from build123d import *

# Parameters (mm, degrees)
F0_W     = 50.8
F0_H     = 400.05
F0_W_2   = 23.167712307
F0_H_2   = 133.35
F0_H_3   = 88.3720067978
F0_H_4   = 368.3754058838
F0_H_5   = 197.3025873184
F0_H_6   = 25.4
F0_H_7   = 431.8
F1_DEPTH = 25.4


with BuildPart() as f1:
    # F0 (on Top) → F1 (new body)
    with BuildSketch(Plane.XY):
        with Locations((0, 200.025)):
            Rectangle(F0_W, F0_H)
        with Locations((-36.9838561535, 466.725)):
            Rectangle(F0_W_2, F0_H_2)
        with Locations((0, 466.725)):
            Rectangle(F0_W, F0_H_2)
        with Locations((36.9838561535, 466.725)):
            Rectangle(F0_W_2, F0_H_2)
        with Locations((-36.9838561535, 577.5860033989)):
            Rectangle(F0_W_2, F0_H_3)
        with Locations((36.9838561535, 577.5860033989)):
            Rectangle(F0_W_2, F0_H_3)
        Polygon((-48.567712307, 621.7720067978), (-25.4, 621.7720067978), (-25.4, 990.1474126816), (-152.4, 990.1474126816), (-152.4, 533.4), (-48.567712307, 533.4), align=None)
        with Locations((0, 805.9597097397)):
            Rectangle(F0_W, F0_H_4)
        Polygon((25.4, 990.1474126816), (25.4, 621.7720067978), (48.567712307, 621.7720067978), (48.567712307, 533.4), (152.4, 533.4), (152.4, 990.1474126816), align=None)
        with Locations((0, 1088.7987063408)):
            Rectangle(F0_W, F0_H_5)
        Polygon((-196.85, 1187.45), (-25.4, 1187.45), (-25.4, 1212.85), (-196.85, 1212.85), (-196.85, 1384.3), (-222.25, 1384.3), (-222.25, 1149.35), (-196.85, 1149.35), align=None)
        with Locations((0, 1200.15)):
            Rectangle(F0_W, F0_H_6)
        Polygon((25.4, 1212.85), (25.4, 1187.45), (196.85, 1187.45), (196.85, 1149.35), (222.25, 1149.35), (222.25, 1384.3), (196.85, 1384.3), (196.85, 1212.85), align=None)
        with Locations((0, 1428.75)):
            Rectangle(F0_W, F0_H_7)
        with Locations((0, 577.5860033989)):
            Rectangle(F0_W, F0_H_3)
    extrude(amount=F1_DEPTH)


solid = f1.part
Read the model definition and answer for the solid it produces. Units are mm, in the model's axes. Coordinates: 2 decimals unless noted, no trailing zeros. Write each loop counter-clockwise with the first axis right and the second up, starting at its lowest first coordinate (ties: lowest second). Pieces come first, ordered by that corner, then holes. Notation, with made-up numbers: (-36.5, -19) -> (15.5, -19) arc R35 ccw to (15.5, 17) -> close; hole circle Ø2 at (79.5, -9.5). An arc over 180 degrees is marked (long way). Return JSON: item names as keys, results as strings.
(1) The part is cut by section D-D on y = 606.5. Give the vertices of the cut face in (x, z), then the cut area to 3 significant figures.
Answers below:
{"outline": "(-152.4, 0) -> (152.4, 0) -> (152.4, 25.4) -> (-152.4, 25.4) -> close", "area": "7,740 mm^2"}
(2) Each of these flat-tipped pins is pushed along its axis until it touches: P1, Ø7.5, axis at y = 752.5, z = 15, coming from the -X side; P2, Ø7, axis at x = -40, z = 16, coming from the -Y side; P3, Ø1.5, axis at y = 528.5, z = 13.5, coming from the -X side. Where does it stop, or does it pass through?
Answers below:
{"P1": "x = -152.4", "P2": "y = 400.05", "P3": "x = -48.57"}
(3) The part is cut by section A-A on x = 86. Give the vertices of the cut face in (y, z).
Answers below:
{"outline": "(533.4, 0) -> (990.15, 0) -> (990.15, 25.4) -> (533.4, 25.4) -> close; (1187.45, 0) -> (1212.85, 0) -> (1212.85, 25.4) -> (1187.45, 25.4) -> close"}
(4) The part is cut by section B-B on y = 1308.5. Give the vertices of the cut face in (x, z).
Answers below:
{"outline": "(-222.25, 0) -> (-196.85, 0) -> (-196.85, 25.4) -> (-222.25, 25.4) -> close; (-25.4, 0) -> (25.4, 0) -> (25.4, 25.4) -> (-25.4, 25.4) -> close; (196.85, 0) -> (222.25, 0) -> (222.25, 25.4) -> (196.85, 25.4) -> close"}
(5) Consider line 1 along X through (y, z) = (1383, 5.25); line 2 along Y through (x, z) = (42, 22.5); line 3 along Y through (x, z) = (133, 3.5). Determine where each line is inside the solid, lowest interval first. Write a range as from..to.
Answers below:
{"line 1": "-222.25..-196.85, -25.4..25.4, 196.85..222.25", "line 2": "400.05..990.15, 1187.45..1212.85", "line 3": "533.4..990.15, 1187.45..1212.85"}
